Here's how the part is built. I have some questions about the finished solid (model axes, mm). A direction names the side the tool comes from. Give positions to 0.01 mm unless a question says otherwise; leave off trailing zeros. Order: outer loops, then holes, each group sorted by start corner. A loop starts at its lowest first (then second) coordinate and runs counter-clockwise, first axis right, second up.
from build123d import *
from build123d.topology import SkipClean

# Parameters (mm, degrees)
SKETCH1_R                = 1.4
SKETCH1_R_2              = 13.25
BOSS_EXTRUDE1_DEPTH      = 3
SKETCH3_R                = 18.25
SKETCH3_R_2              = 15.25
BOSS_EXTRUDE2_DEPTH      = 15
BOSS_EXTRUDE4_DEPTH      = 2
BOSS_EXTRUDE5_DEPTH      = 3
CUT_EXTRUDE1_START       = -3
CUT_EXTRUDE1_OUTLINE_R   = 1.75
CUT_EXTRUDE1_OUTLINE_R_2 = 1.4
CUT_EXTRUDE1_DEPTH       = 3


# Read off the part's stored shape, not the designer's step: Cut-Extrude1
with BuildPart() as part:
    # Sketch1 → Boss-Extrude1 (new body)
    with BuildSketch(Plane.XY):
        with BuildLine():
            ThreePointArc((22.025, 11.45), (20.896729165, 14.329079757), (18.112740296, 15.675))
            Line((18.112740296, 15.675), (9.346489983, 15.675))
            ThreePointArc((9.346489983, 15.675), (0, 18.25), (-9.346489983, 15.675))
            Line((-9.346489983, 15.675), (-18.112740296, 15.675))
            ThreePointArc((-18.112740296, 15.675), (-20.896729165, 14.329079757), (-22.025, 11.45))
            Line((-22.025, 11.45), (-22.025, -11.45))
            ThreePointArc((-22.025, -11.45), (-20.896729165, -14.329079757), (-18.112740296, -15.675))
            Line((-18.112740296, -15.675), (-9.346489983, -15.675))
            ThreePointArc((-9.346489983, -15.675), (0, -18.25), (9.346489983, -15.675))
            Line((9.346489983, -15.675), (18.112740296, -15.675))
            ThreePointArc((18.112740296, -15.675), (20.896729165, -14.329079757), (22.025, -11.45))
            Line((22.025, -11.45), (22.025, 11.45))
        make_face()
        with Locations((17.7875, -11.45)):
            Circle(SKETCH1_R, mode=Mode.SUBTRACT)
        with Locations((17.7875, 11.45)):
            Circle(SKETCH1_R, mode=Mode.SUBTRACT)
        with Locations((-17.7875, 11.45)):
            Circle(SKETCH1_R, mode=Mode.SUBTRACT)
        with Locations((-17.7875, -11.45)):
            Circle(SKETCH1_R, mode=Mode.SUBTRACT)
        Circle(SKETCH1_R_2, mode=Mode.SUBTRACT)
    extrude(amount=BOSS_EXTRUDE1_DEPTH)

    # Sketch3 → Boss-Extrude2 (add)
    with BuildSketch(Plane.XY.offset(3)):
        with Locations(Location((0, 0, 0), (0, 0, 120.806241835))):
            Circle(SKETCH3_R)
        Circle(SKETCH3_R_2, mode=Mode.SUBTRACT)
    extrude(amount=BOSS_EXTRUDE2_DEPTH)

    # Sketch5 → Boss-Extrude4 (add)
    with SkipClean():  # the faces are left unmerged after this step: merging them gives an invalid solid
        with BuildSketch(Plane.XY.offset(3)):
            with BuildLine():
                ThreePointArc((-15.25, -5.3e-08), (-15.241792239, -0.500269278), (-15.217177794, -1))
                Line((-15.217177794, -1), (-13.212210262, -1))
                ThreePointArc((-13.212210262, -1), (-13.25, 0), (-13.212210262, 1))
                Line((-13.212210262, 1), (-15.217177794, 1))
                ThreePointArc((-15.217177794, 1), (-15.24179224, 0.500269225), (-15.25, -5.3e-08))
            make_face()
            with BuildLine():
                Line((13.212210262, -1), (15.217177794, -1))
                ThreePointArc((15.217177794, -1), (15.24179224, -0.500269252), (15.25, 0))
                ThreePointArc((15.25, 0), (15.24179224, 0.500269252), (15.217177794, 1))
                Line((15.217177794, 1), (13.212210262, 1))
                ThreePointArc((13.212210262, 1), (13.240549195, 0.500356889), (13.25, 0))
                ThreePointArc((13.25, 0), (13.240549195, -0.500356889), (13.212210262, -1))
            make_face()
        extrude(amount=BOSS_EXTRUDE4_DEPTH)

    # Sketch6 → Boss-Extrude5 (add)
    with SkipClean():  # the faces are left unmerged after this step: merging them gives an invalid solid
        with BuildSketch(Plane(origin=(0, 0, 0), x_dir=(-1, 0, 0), z_dir=(0, 0, -1))):
            with BuildLine():
                ThreePointArc((-5.5, -12.054563451), (-4.028545362, -12.622730381), (-2.5, -13.01201368))
                Line((-2.5, -13.01201368), (-2.5, 13.01201368))
                ThreePointArc((-2.5, 13.01201368), (-4.028545362, 12.622730381), (-5.5, 12.054563451))
                Line((-5.5, 12.054563451), (-5.5, -12.054563451))
            make_face()
            with BuildLine():
                Line((2.5, 13.01201368), (2.5, -13.01201368))
                ThreePointArc((2.5, -13.01201368), (4.028545362, -12.622730381), (5.5, -12.054563451))
                Line((5.5, -12.054563451), (5.5, 12.054563451))
                ThreePointArc((5.5, 12.054563451), (4.028545362, 12.622730381), (2.5, 13.01201368))
            make_face()
        extrude(amount=-BOSS_EXTRUDE5_DEPTH)

    # Cut-Extrude1 outline → Cut-Extrude1 (cut)
    # profile 1 of 4: a face of its own
    with SkipClean():  # the faces are left unmerged after this step: merging them gives an invalid solid
        with BuildSketch(Plane.XY.offset(3).offset(CUT_EXTRUDE1_START)):
            with Locations((-17.7875, 11.45)):
                Circle(CUT_EXTRUDE1_OUTLINE_R)
            with Locations((-17.7875, 11.45)):
                Circle(CUT_EXTRUDE1_OUTLINE_R_2, mode=Mode.SUBTRACT)
        # profile 2 of 4: a face of its own
        with BuildSketch(Plane.XY.offset(3).offset(CUT_EXTRUDE1_START)):
            with Locations((-17.7875, -11.45)):
                Circle(CUT_EXTRUDE1_OUTLINE_R)
            with Locations((-17.7875, -11.45)):
                Circle(CUT_EXTRUDE1_OUTLINE_R_2, mode=Mode.SUBTRACT)
        # profile 3 of 4: a face of its own
        with BuildSketch(Plane.XY.offset(3).offset(CUT_EXTRUDE1_START)):
            with Locations((17.7875, -11.45)):
                Circle(CUT_EXTRUDE1_OUTLINE_R)
            with Locations((17.7875, -11.45)):
                Circle(CUT_EXTRUDE1_OUTLINE_R_2, mode=Mode.SUBTRACT)
        # profile 4 of 4: a face of its own
        with BuildSketch(Plane.XY.offset(3).offset(CUT_EXTRUDE1_START)):
            with Locations((17.7875, 11.45)):
                Circle(CUT_EXTRUDE1_OUTLINE_R)
            with Locations((17.7875, 11.45)):
                Circle(CUT_EXTRUDE1_OUTLINE_R_2, mode=Mode.SUBTRACT)
        extrude(amount=CUT_EXTRUDE1_DEPTH, mode=Mode.SUBTRACT)


solid = part.part
Q1. For faces 1 (the face through (14, -15.675, 1)), 2 (the face through (-14, 1, 4)), 3 (the face through (-0.04, -13.25, 1.48)), 4 (the face through (-14, -15.675, 1)), which set-ups out of +Z, -Z, +X, -X, +Y, -Y let a thin tool reach every point of the face, with its end or its side?
Filled sheet:
face 1: +Z, -Z, +X, -Y
face 2: +Z
face 3: +Z, -Z
face 4: +Z, -Z, -X, -Y
Q2. I need wall thicknesses on L1, parallel to Y at x = 0, z = 11; L2, parallel to X at y = -0.5, z = 10.5; L3, parallel to X at y = -11, z = 2.25 (3 decimals). Which ranges of each line are inside material? Lowest first, please.
Filled sheet:
L1: y = -18.25 to -15.25, 15.25 to 18.25
L2: x = -18.24 to -15.24, 15.24 to 18.24
L3: x = -22.025 to -19.479, -16.096 to -7.387, -5.5 to -2.5, 2.5 to 5.5, 7.387 to 16.096, 19.479 to 22.025
Q3. If we section it at C-C on y = -7: List the corners of the cut face in (x, z) for me (3 decimals).
Filled sheet:
outline: (-22.025, 0) - (-11.25, 0) - (-11.25, 3) - (-13.549, 3) - (-13.549, 18) - (-16.854, 18) - (-16.854, 3) - (-22.025, 3) - close; (-5.5, 0) - (-2.5, 0) - (-2.5, 3) - (-5.5, 3) - close; (2.5, 0) - (5.5, 0) - (5.5, 3) - (2.5, 3) - close; (11.25, 0) - (22.025, 0) - (22.025, 3) - (16.854, 3) - (16.854, 18) - (13.549, 18) - (13.549, 3) - (11.25, 3) - close
Q4. If we section it at D-D on z = 14: List the corners of the cut face in (x, y) for me (3 decimals), plus the area to 3 significant figures.
Filled sheet:
outline: circle Ø36.5 at (0, 0); hole circle Ø30.5 at (0, 0)
area: 316 mm2
Q5. If we section it at A-A on x = 0: List the corners of the cut face in (y, z) for me.
Filled sheet:
outline: (-18.25, 0) - (-13.25, 0) - (-13.25, 3) - (-15.25, 3) - (-15.25, 18) - (-18.25, 18) - close; (13.25, 0) - (18.25, 0) - (18.25, 18) - (15.25, 18) - (15.25, 3) - (13.25, 3) - close
Q6. I'm going to push flat-ended pins straight in: P1, Ø1, axis at x = 14.5, z = 4, coming from the -Y side; P2, Ø3.5, axis at x = -15.5, z = 2, coming from the +Y side (3 decimals); P3, Ø0.9, axis at x = 15.5, z = 2, coming from the -Y side (3 decimals); P4, Ø3, axis at x = -17.79, y = -11.45, coming from the -Z side. Where does each tip first touch, or does it pass through?
Filled sheet:
P1: stops at y = -11.71
P2: stops at y = 15.675
P3: stops at y = -15.675
P4: passes through
Q7. If we section it at B-B on z = 1.5: Give the number of separate pieces and of enclosed holes in the cut face, plus the area to 3 significant figures.
Filled sheet:
separate pieces: 1
enclosed holes: 7
area: 992 mm2
Q8. Thinking about a two-plate mould opening in Y: for faces 5 (the face through (20.87, -14.36, 1.48)), 6 (the face through (5.5, 0, 1)), 7 (the face through (-19, 0, 3)), which applies, released by +Y, released by -Y, zero draft, split by the parting line, or undercut?
Filled sheet:
face 5: released by -Y
face 6: undercut
face 7: zero draft
